```python
from build123d import *

# Parameters (mm, degrees)
F1_W     = 499.5
F1_H     = 1199.5
F1_R     = 2.5
F2_DEPTH = 19


with BuildPart() as f2:
    # F1 (on Front) → F2 (new body)
    with BuildSketch(Plane.XZ):
        with Locations((249.75, 990.25)):
            Rectangle(F1_W, F1_H)
        with Locations((50, 661.2)):
            Circle(F1_R, mode=Mode.SUBTRACT)
        with BuildLine():
            Line((85, 603), (165, 603))
            ThreePointArc((165, 603), (168.5355339059, 601.5355339059), (170, 598))
            Line((170, 598), (170, 588))
            ThreePointArc((170, 588), (168.5355339059, 584.4644660941), (165, 583))
            Line((165, 583), (85, 583))
            ThreePointArc((85, 583), (81.4644660941, 584.4644660941), (80, 588))
            Line((80, 588), (80, 598))
            ThreePointArc((80, 598), (81.4644660941, 601.5355339059), (85, 603))
        make_face(mode=Mode.SUBTRACT)
        with Locations((200, 661.2)):
            Circle(F1_R, mode=Mode.SUBTRACT)
        with Locations((300, 661.2)):
            Circle(F1_R, mode=Mode.SUBTRACT)
        with BuildLine():
            Line((335, 603), (415, 603))
            ThreePointArc((415, 603), (418.5355339059, 601.5355339059), (420, 598))
            Line((420, 598), (420, 588))
            ThreePointArc((420, 588), (418.5355339059, 584.4644660941), (415, 583))
            Line((415, 583), (335, 583))
            ThreePointArc((335, 583), (331.4644660941, 584.4644660941), (330, 588))
            Line((330, 588), (330, 598))
            ThreePointArc((330, 598), (331.4644660941, 601.5355339059), (335, 603))
        make_face(mode=Mode.SUBTRACT)
        with Locations((450, 661.2)):
            Circle(F1_R, mode=Mode.SUBTRACT)
        with Locations((125, 848)):
            Circle(F1_R, mode=Mode.SUBTRACT)
        with BuildLine():
            Line((85, 953), (165, 953))
            ThreePointArc((165, 953), (168.5355339059, 951.5355339059), (170, 948))
            Line((170, 948), (170, 938))
            ThreePointArc((170, 938), (168.5355339059, 934.4644660941), (165, 933))
            Line((165, 933), (85, 933))
            ThreePointArc((85, 933), (81.4644660941, 934.4644660941), (80, 938))
            Line((80, 938), (80, 948))
            ThreePointArc((80, 948), (81.4644660941, 951.5355339059), (85, 953))
        make_face(mode=Mode.SUBTRACT)
        with Locations((375, 848)):
            Circle(F1_R, mode=Mode.SUBTRACT)
        with BuildLine():
            Line((335, 953), (415, 953))
            ThreePointArc((415, 953), (418.5355339059, 951.5355339059), (420, 948))
            Line((420, 948), (420, 938))
            ThreePointArc((420, 938), (418.5355339059, 934.4644660941), (415, 933))
            Line((415, 933), (335, 933))
            ThreePointArc((335, 933), (331.4644660941, 934.4644660941), (330, 938))
            Line((330, 938), (330, 948))
            ThreePointArc((330, 948), (331.4644660941, 951.5355339059), (335, 953))
        make_face(mode=Mode.SUBTRACT)
        with Locations((50, 1011.2)):
            Circle(F1_R, mode=Mode.SUBTRACT)
        with Locations((200, 1011.2)):
            Circle(F1_R, mode=Mode.SUBTRACT)
        with Locations((125, 1198)):
            Circle(F1_R, mode=Mode.SUBTRACT)
        with Locations((300, 1011.2)):
            Circle(F1_R, mode=Mode.SUBTRACT)
        with Locations((450, 1011.2)):
            Circle(F1_R, mode=Mode.SUBTRACT)
        with Locations((375, 1198)):
            Circle(F1_R, mode=Mode.SUBTRACT)
        with Locations((50, 1361.2)):
            Circle(F1_R, mode=Mode.SUBTRACT)
        with BuildLine():
            ThreePointArc((170, 1288), (168.5355339059, 1284.4644660941), (165, 1283))
            Line((165, 1283), (85, 1283))
            ThreePointArc((85, 1283), (81.4644660941, 1284.4644660941), (80, 1288))
            Line((80, 1288), (80, 1298))
            ThreePointArc((80, 1298), (81.4644660941, 1301.5355339059), (85, 1303))
            Line((85, 1303), (165, 1303))
            ThreePointArc((165, 1303), (168.5355339059, 1301.5355339059), (170, 1298))
            Line((170, 1298), (170, 1288))
        make_face(mode=Mode.SUBTRACT)
        with Locations((200, 1361.2)):
            Circle(F1_R, mode=Mode.SUBTRACT)
        with Locations((125, 1548)):
            Circle(F1_R, mode=Mode.SUBTRACT)
        with Locations((300, 1361.2)):
            Circle(F1_R, mode=Mode.SUBTRACT)
        with BuildLine():
            Line((335, 1303), (415, 1303))
            ThreePointArc((415, 1303), (418.5355339059, 1301.5355339059), (420, 1298))
            Line((420, 1298), (420, 1288))
            ThreePointArc((420, 1288), (418.5355339059, 1284.4644660941), (415, 1283))
            Line((415, 1283), (335, 1283))
            ThreePointArc((335, 1283), (331.4644660941, 1284.4644660941), (330, 1288))
            Line((330, 1288), (330, 1298))
            ThreePointArc((330, 1298), (331.4644660941, 1301.5355339059), (335, 1303))
        make_face(mode=Mode.SUBTRACT)
        with Locations((450, 1361.2)):
            Circle(F1_R, mode=Mode.SUBTRACT)
        with Locations((375, 1548)):
            Circle(F1_R, mode=Mode.SUBTRACT)
    extrude(amount=F2_DEPTH)


with BuildPart() as f2_1:
    # F3: moved
    add(f2.part.moved(Location((0, 0, -390.5))))


solid = f2_1.part
```
Verification items for the finished model (mm, model axes). Round coordinates to 2 decimals unless told otherwise and drop trailing zeros. Put each result on its own line as item: value. Start each with the question number.
(1) Section check A-A (y = -9.25). State how many separate pieces and enclosed holes the cut face has, then the cut area to 3 significant figures.
(2) Material ranges on line 1 along Z through (x, y) = (50, -14.5); line 2 along Z through (x, y) = (112, -16); line 3 along X through (y, z) = (-13, 620.7), recorded low to high.
(3) Depth check by flat-ended pin: pin 1 Ø4.5 at (x, z) = (300, 270.7) entering from -Y. Enter the tip coordinate at first touch or a pass-through.
Completed:
1. separate pieces: 1
1. enclosed holes: 24
1. area: 588,000 mm2
2. line 1: z = 0 to 268.2, 273.2 to 618.2, 623.2 to 968.2, 973.2 to 1199.5
2. line 2: z = 0 to 192.5, 212.5 to 542.5, 562.5 to 892.5, 912.5 to 1199.5
2. line 3: x = 0 to 47.5, 52.5 to 197.5, 202.5 to 297.5, 302.5 to 447.5, 452.5 to 499.5
3. pin 1: passes through
